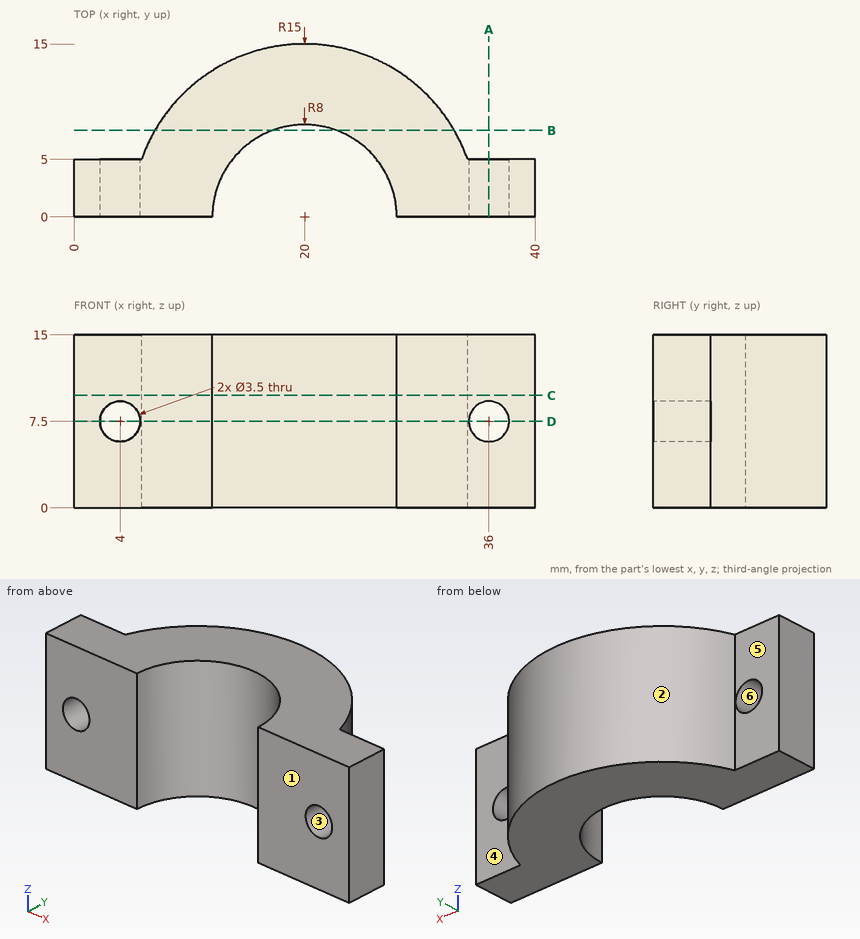
Print and shaded views of the part. All mm, measured from the part's lowest x, y and z. A direction names the side the tool comes from. Coordinates: 2 decimals unless noted, no trailing zeros. Write each loop counter-clockwise with the first axis right and the second up, starting at its lowest first coordinate (ties: lowest second). Pieces come first, ordered by that corner, then holes.
(1) Two-plate mould, pull along X, no slides. Class the marked faces 1, 2 and 3: +X half, -X half, draft (parallel to the pull), parting line (faces both ways), or undercut.
(2) Cut at C-C, the plane z = 9.75. List the corners of the cut face in (x, y).
(3) Cut at A-A, the plane x = 36. List the corners of the cut face in (y, z).
(4) Flat gauge pins, fed straight in: pin 1 (1.5 mm diameter, centred on x = 18, z = 7.5, fed in from -Y); pin 2 (1.5 mm diameter, centred on x = 7.5, y = 12.5, fed in from +Z); pin 3 (3 mm diameter, centred on x = 11, z = 5, fed in from +Y); pin 4 (4.5 mm diameter, centred on x = 2, z = 11, fed in from +Y). Where does each tip first touch, or does it go through?
(5) 3-axis set-ups, long thin cutter, end or side, ignore diameter. For the marked faces 4, 5 and 6: which of +Z, -Z, +X, -X, +Y, -Y reach the whole face in a straight line?
(6) Drill centre lines: probe 1 along Z at (x, y) = (4, 2.7); probe 2 along X at (y, z) = (4.75, 6); probe 3 along X at (y, z) = (3.25, 8). Where is each one in solid material? Low to high.
(7) Cut at D-D, the plane z = 7.5. List the corners of the cut face in (x, y).
(8) Cut at B-B, the plane y = 7.5. List the corners of the cut face in (x, z).
Geometry says:
1. face 1: draft
1. face 2: parting line
1. face 3: undercut
2. outline: (0, 0) - (12, 0) arc R8 cw to (28, 0) - (40, 0) - (40, 5) - (34.14, 5) arc R15 ccw to (5.86, 5) - (0, 5) - close
3. outline: (0, 0) - (5, 0) - (5, 5.75) - (0, 5.75) - close; (0, 9.25) - (5, 9.25) - (5, 15) - (0, 15) - close
4. pin 1: stops at y = 7.51
4. pin 2: passes through
4. pin 3: stops at y = 12.99
4. pin 4: stops at y = 5
5. face 4: +Z, -Z, +X, +Y
5. face 5: +Z, -Z, -X, +Y
5. face 6: +Y, -Y
6. probe 1: z = 0 to 5.75, 9.25 to 15
6. probe 2: x = 0 to 3.1, 4.9 to 13.56, 26.44 to 35.1, 36.9 to 40
6. probe 3: x = 0 to 2.32, 5.68 to 12.69, 27.31 to 34.32, 37.68 to 40
7. outline: (0, 0) - (2.25, 0) - (2.25, 5) - (0, 5) - close; (5.75, 0) - (12, 0) arc R8 cw to (28, 0) - (34.25, 0) - (34.25, 5) - (34.14, 5) arc R15 ccw to (5.86, 5) - (5.75, 5) - close; (37.75, 0) - (40, 0) - (40, 5) - (37.75, 5) - close
8. outline: (7.01, 0) - (17.22, 0) - (17.22, 15) - (7.01, 15) - close; (22.78, 0) - (32.99, 0) - (32.99, 15) - (22.78, 15) - close
